```python
from build123d import *

# Parameters (mm, degrees)
SKETCH2_W            = 370
SKETCH2_H            = 690
SKETCH2_W_2          = 270
SKETCH2_H_2          = 590
BOSS_EXTRUDE1_DEPTH  = 20
CHAMFER1_SIZE        = 20
SKETCH10_W           = 370
SKETCH10_H           = 690
BOSS_EXTRUDE6_DEPTH  = 20
CUT_EXTRUDE3_DEPTH   = 784.964284901
SKETCH11_W           = 30
SKETCH11_H           = 30
BOSS_EXTRUDE7_DEPTH  = 130
SKETCH13_W           = 200
SKETCH13_H           = 50
CUT_EXTRUDE4_DEPTH   = 20
BOSS_EXTRUDE11_DEPTH = 690
BOSS_EXTRUDE15_DEPTH = 40
SKETCH21_W           = 0.428939058
SKETCH21_H           = 0.058642304
SKETCH21_W_2         = 75.212075904
SKETCH21_H_2         = 45.043559158
CUT_EXTRUDE6_DEPTH   = 17
BOSS_EXTRUDE16_DEPTH = 250


with BuildPart() as part:
    # Sketch2 → Boss-Extrude1 (new body)
    with BuildSketch(Plane(origin=(0, 0, 0), x_dir=(1, 0, 0), z_dir=(0, 1, 0))):
        with Locations((185, 345)):
            Rectangle(SKETCH2_W, SKETCH2_H)
        with Locations((185, 345)):
            Rectangle(SKETCH2_W_2, SKETCH2_H_2, mode=Mode.SUBTRACT)
    extrude(amount=BOSS_EXTRUDE1_DEPTH)

    # Chamfer1
    chamfer1_edges = [part.edges().sort_by_distance(p)[0] for p in [
        (185, 0, -640),
        (320, 0, -345),
        (185, 0, -50),
        (50, 0, -345),
    ]]
    chamfer(chamfer1_edges, length=CHAMFER1_SIZE - 0.0001)  # a hair under: the kernel refuses the full size

    # Sketch10 → Boss-Extrude6 (add)
    with BuildSketch(Plane.XZ):
        with Locations((185, -345)):
            Rectangle(SKETCH10_W, SKETCH10_H)
    extrude(amount=BOSS_EXTRUDE6_DEPTH)

    # Sketch4 → Cut-Extrude3 (cut, through all)
    with BuildSketch(Plane(origin=(0, 20, 0), x_dir=(1, 0, 0), z_dir=(0, 1, 0))):
        with BuildLine():
            ThreePointArc((320, 615), (337.67766953, 622.32233047), (345, 640))
            ThreePointArc((345, 640), (320, 665), (295, 640))
            Line((295, 640), (320, 640))
            Line((320, 640), (320, 615))
        make_face()
        with BuildLine():
            Line((320, 640), (295, 640))
            ThreePointArc((295, 640), (302.32233047, 622.32233047), (320, 615))
            Line((320, 615), (320, 640))
        make_face()
        with BuildLine():
            Line((50, 640), (75, 640))
            ThreePointArc((75, 640), (32.32233047, 657.67766953), (50, 615))
            Line((50, 615), (50, 640))
        make_face()
        with BuildLine():
            ThreePointArc((50, 615), (67.67766953, 622.32233047), (75, 640))
            Line((75, 640), (50, 640))
            Line((50, 640), (50, 615))
        make_face()
        with BuildLine():
            Line((50, 320), (50, 370))
            ThreePointArc((50, 370), (25, 345), (50, 320))
        make_face()
        with BuildLine():
            ThreePointArc((75, 345), (67.67766953, 362.67766953), (50, 370))
            Line((50, 370), (50, 320))
            ThreePointArc((50, 320), (67.67766953, 327.32233047), (75, 345))
        make_face()
        with BuildLine():
            Line((50, 50), (50, 75))
            ThreePointArc((50, 75), (32.32233047, 32.32233047), (75, 50))
            Line((75, 50), (50, 50))
        make_face()
        with BuildLine():
            ThreePointArc((75, 50), (67.67766953, 67.67766953), (50, 75))
            Line((50, 75), (50, 50))
            Line((50, 50), (75, 50))
        make_face()
        with BuildLine():
            Line((320, 50), (320, 75))
            ThreePointArc((320, 75), (302.32233047, 67.67766953), (295, 50))
            Line((295, 50), (320, 50))
        make_face()
        with BuildLine():
            ThreePointArc((345, 50), (337.67766953, 67.67766953), (320, 75))
            Line((320, 75), (320, 50))
            Line((320, 50), (295, 50))
            ThreePointArc((295, 50), (320, 25), (345, 50))
        make_face()
        with BuildLine():
            Line((320, 320), (320, 370))
            ThreePointArc((320, 370), (295, 345), (320, 320))
        make_face()
        with BuildLine():
            ThreePointArc((345, 345), (337.67766953, 362.67766953), (320, 370))
            Line((320, 370), (320, 320))
            ThreePointArc((320, 320), (337.67766953, 327.32233047), (345, 345))
        make_face()
    extrude(amount=-CUT_EXTRUDE3_DEPTH, mode=Mode.SUBTRACT)

    # Sketch11 → Boss-Extrude7 (add)
    with BuildSketch(Plane.XZ.offset(20)):
        with Locations((15, -15)):
            Rectangle(SKETCH11_W, SKETCH11_H)
        with Locations((355, -15)):
            Rectangle(SKETCH11_W, SKETCH11_H)
        with Locations((15, -675)):
            Rectangle(SKETCH11_W, SKETCH11_H)
        with Locations((355, -675)):
            Rectangle(SKETCH11_W, SKETCH11_H)
    extrude(amount=BOSS_EXTRUDE7_DEPTH)

    # Sketch13 → Cut-Extrude4 (cut)
    with BuildSketch(Plane(origin=(0, 20, 0), x_dir=(1, 0, 0), z_dir=(0, 1, 0))):
        with Locations((180, 665)):
            Rectangle(SKETCH13_W, SKETCH13_H)
    extrude(amount=-CUT_EXTRUDE4_DEPTH, mode=Mode.SUBTRACT)

    # Sketch14 → Boss-Extrude11 (add)
    with BuildSketch(Plane.XY):
        Polygon((30, -52.106305214), (300, -71.063052139), (300, -91.063052139), (30, -72.106305214), align=None)
    extrude(amount=-BOSS_EXTRUDE11_DEPTH)

    # Sketch19 → Boss-Extrude15 (add)
    with BuildSketch(Plane(origin=(300, 0, 0), x_dir=(0, 0, -1), z_dir=(1, 0, 0))):
        Polygon((0, -71.063052139), (690, -131.063052139), (690, -151.063052139), (0, -91.063052139), align=None)
    extrude(amount=BOSS_EXTRUDE15_DEPTH)

    # Sketch21 → Cut-Extrude6 (cut)
    with BuildSketch(Plane.XZ.offset(150)):
        with Locations((372.006097864, -651.747092541)):
            Rectangle(SKETCH21_W, SKETCH21_H)
        with Locations((331.793311609, -674.26887212)):
            Rectangle(SKETCH21_W_2, SKETCH21_H_2)
    extrude(amount=CUT_EXTRUDE6_DEPTH, mode=Mode.SUBTRACT)

    # Sketch22 → Boss-Extrude16 (add)
    with BuildSketch(Plane(origin=(0, 0, -690), x_dir=(-1, 0, 0), z_dir=(0, 0, -1))):
        with BuildLine():
            Line((-305, -131.063052139), (-300, -131.063052139))
            Line((-300, -131.063052139), (-300, -150))
            Line((-300, -150), (-340, -150))
            Line((-340, -150), (-340, -131.063052139))
            Line((-340, -131.063052139), (-335, -131.063052139))
            ThreePointArc((-335, -131.063052139), (-320, -146.063052139), (-305, -131.063052139))
        make_face()
    extrude(amount=BOSS_EXTRUDE16_DEPTH)


solid = part.part
```
Input: part model. Units: mm. Frame: model coordinates. A direction names the side the tool comes from. Round coordinates to 2 decimals unless told otherwise and drop trailing zeros. Loops run counter-clockwise (first coordinate to the right, second up) from the corner with the lowest first, then second, coordinate; pieces in that order, holes last. Notation, with made-up numbers: (-28, 51) -> (8, 51) arc R20 cw to (8, 88) -> close; hole circle Ø11 at (73.25, -26). An arc over 180 degrees is marked (long way). Use one line per item in the form item = value. Start each with the question number.
Item 1: Contact query for flat-ended pins moving along their axis: pin 1 Ø6 at (y, z) = (-77, -694) entering from -X; pin 2 Ø15 at (y, z) = (-139, -848.5) entering from +X; pin 3 Ø2 at (y, z) = (-56.5, -652.5) entering from -X; pin 4 Ø4.5 at (x, y) = (320.5, -138) entering from -Z. Output: stop coordinate, or through.
Item 2: Mould query, pull axis X, two halves, no side actions, for faces 1 (the face through (340, -141, -813)), 2 (the face through (355, -84, -660)), 3 (the face through (290, 10, -650)). Classes: pulls with the +X half, pulls with the -X half, needs draft (parallel to the pull), parting line crosses it, or undercut.
Item 3: Section query D-D on z = -461.5. Count the separate pieces of the cut face and the enclosed holes in it, then the cut area to 3 significant figures.
Item 4: Set-up query: faces 4 (the face through (183, 0, -365)), 5 (the face through (30, -36, -675)), 6 (the face through (80, 10, -670)). Return all of +Z, -Z, +X, -X, +Y, -Y with unobstructed straight access to the full face (end or side cutting, diameter ignored); none if empty.
Item 5: Section query B-B on y = -106.5. Return the cut outline in (x, z).
Item 6: Material intervals for L1, parallel to Z at x = 50, y = -10; L2, parallel to X at y = 8, z = -50; L3, parallel to Z at x = 350, y = -89.5, sorted ascending. Write a range as from..to.
Ans:
q1.pin_1 = through
q1.pin_2 = 340
q1.pin_3 = 30
q1.pin_4 = -690
q2.face_1 = pulls with the +X half
q2.face_2 = needs draft
q2.face_3 = undercut
q3.separate_pieces = 3
q3.enclosed_holes = 0
q3.area = 15,200 mm^2
q4.face_4 = none
q4.face_5 = +Z, -Z
q4.face_6 = -Z, +Y
q5.outline = (0, -690) -> (30, -690) -> (30, -660) -> (0, -660) -> close; (0, -30) -> (30, -30) -> (30, 0) -> (0, 0) -> close; (300, -407.52) -> (340, -407.52) -> (340, -177.52) -> (300, -177.52) -> close; (340, -690) -> (370, -690) -> (370, -660) -> (340, -660) -> close; (340, -30) -> (370, -30) -> (370, 0) -> (340, 0) -> close
q6.L1 = -690..-665, -615..-370, -320..-75, -25..0
q6.L2 = 0..25, 345..370
q6.L3 = -690..-660, -30..0
